```python
from build123d import *

# Parameters (mm, degrees)
SKETCH1_W           = 168
SKETCH1_H           = 112
BOSS_EXTRUDE1_DEPTH = 3
SKETCH2_W           = 23
SKETCH2_H           = 28
BOSS_EXTRUDE2_DEPTH = 81
SKETCH11_W          = 28
SKETCH11_H          = 23
CUT_EXTRUDE4_DEPTH  = 12
SKETCH13_W          = 2.5
SKETCH13_H          = 33.689893656
CUT_EXTRUDE5_DEPTH  = 12
SKETCH17_RX         = 11
SKETCH17_RY         = 10
CUT_EXTRUDE6_DEPTH  = 40
SKETCH18_R          = 17
BOSS_EXTRUDE3_DEPTH = 18
SKETCH19_R          = 14
CUT_EXTRUDE7_DEPTH  = 18
SKETCH20_W          = 20
SKETCH20_H          = 25.807879142
CUT_EXTRUDE8_DEPTH  = 18


with BuildPart() as part:
    # Sketch1 → Boss-Extrude1 (new body)
    with BuildSketch(Plane(origin=(0, 0, 0), x_dir=(1, 0, 0), z_dir=(0, 1, 0))):
        Rectangle(SKETCH1_W, SKETCH1_H)
    extrude(amount=BOSS_EXTRUDE1_DEPTH)

    # Sketch2 → Boss-Extrude2 (add)
    with BuildSketch(Plane(origin=(0, 3, 0), x_dir=(1, 0, 0), z_dir=(0, 1, 0))):
        with Locations((-56.5, 30.5)):
            Rectangle(SKETCH2_W, SKETCH2_H)
    boss_extrude2 = extrude(amount=BOSS_EXTRUDE2_DEPTH)

    # Mirror1: Boss-Extrude2 across plane
    add(boss_extrude2.mirror(Plane(origin=(0, 0, 0), x_dir=(0, 0, 1), z_dir=(1, 0, 0))))

    # Sketch11 → Cut-Extrude4 (cut)
    with BuildSketch(Plane(origin=(0, 84, 0), x_dir=(1, 0, 0), z_dir=(0, 1, 0))):
        with Locations((-59, 30.5)):
            Rectangle(SKETCH11_W, SKETCH11_H)
    extrude(amount=-CUT_EXTRUDE4_DEPTH, mode=Mode.SUBTRACT)

    # Sketch13 → Cut-Extrude5 (cut)
    with BuildSketch(Plane(origin=(0, 72, 0), x_dir=(1, 0, 0), z_dir=(0, 1, 0))):
        with Locations((-50, 30.5)):
            Rectangle(SKETCH13_W, SKETCH13_H)
    extrude(amount=CUT_EXTRUDE5_DEPTH, mode=Mode.SUBTRACT)

    # Sketch17 → Cut-Extrude6 (cut)
    with BuildSketch(Plane.ZY.offset(-45)):
        with Locations((-30.5, 84)):
            Ellipse(SKETCH17_RX, SKETCH17_RY)
    extrude(amount=-CUT_EXTRUDE6_DEPTH, mode=Mode.SUBTRACT)

    # Sketch18 → Boss-Extrude3 (add)
    with BuildSketch(Plane(origin=(0, 3, 0), x_dir=(1, 0, 0), z_dir=(0, 1, 0))):
        with Locations(Location((0, -15.5, 0), (0, 0, 90))):
            Circle(SKETCH18_R)
    extrude(amount=BOSS_EXTRUDE3_DEPTH)

    # Sketch19 → Cut-Extrude7 (cut)
    with BuildSketch(Plane(origin=(0, 21, 0), x_dir=(1, 0, 0), z_dir=(0, 1, 0))):
        with Locations(Location((0, -15.5, 0), (0, 0, 270))):
            Circle(SKETCH19_R)
    extrude(amount=-CUT_EXTRUDE7_DEPTH, mode=Mode.SUBTRACT)

    # Sketch20 → Cut-Extrude8 (cut)
    with BuildSketch(Plane(origin=(0, 21, 0), x_dir=(1, 0, 0), z_dir=(0, 1, 0))):
        with Locations((0, -32.5)):
            Rectangle(SKETCH20_W, SKETCH20_H)
    extrude(amount=-CUT_EXTRUDE8_DEPTH, mode=Mode.SUBTRACT)


solid = part.part
```
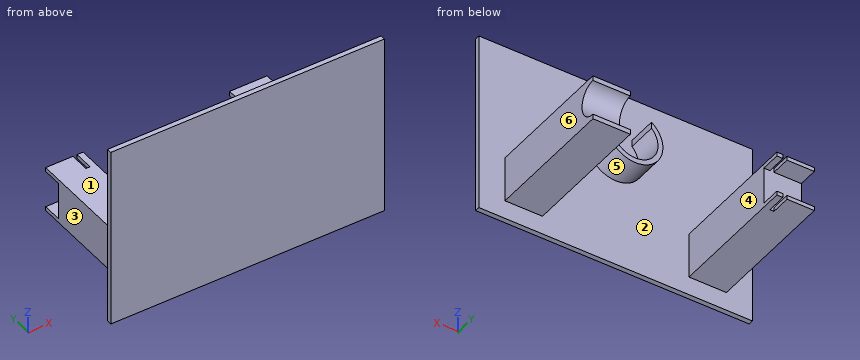
Read the model definition and answer for the solid it produces. Units are mm, in the model's axes. Face numbers are marked on the shaded views. A direction names the side the tool comes from. Round coordinates to 2 decimals unless told otherwise and drop trailing zeros. Write each loop counter-clockwise with the first axis right and the second up, starting at its lowest first coordinate (ties: lowest second). Pieces come first, ordered by that corner, then holes. Notation, with made-up numbers: (-26.5, 65) -> (13.5, 65) arc R26 ccw to (13.5, 101) -> close; hole circle Ø5 at (48, 61.25). An arc over 180 degrees is marked (long way). Answer in a Markdown table with one row per item. Add a question column.
1) Find section B-B, the plane y = 34. Determine the outline of the cut face in (x, z).
2) Find section C-C, the plane z = 15.5. Determine the outline of the cut face in (x, y), and give its area (3 significant figures).
3) Consider line 1 (X direction, y = 62.5, z = -38); line 2 (X direction, y = 12.75, z = 15.5); line 3 (Z direction, x = -65, y = 17). Determine where each line is inside the solid, lowest interval first.
4) Which of the six approach directions +Z, -Z, +X, -X, +Y, -Y give full straight-line access (tool end or side, diameter ignored) to the marked faces 4, 5 and 6?
5) Determine the mould class of the marked faces 1, 2 and 3 for opening direction X: pulls with the +X half, pulls with the -X half, needs draft (parallel to the pull), parting line crosses it, or undercut.
6) Find section D-D, the plane x = -56. Determine the outline of the cut face in (y, z), and give its area (3 significant figures).
7) Given P1, Ø11.5, axis at x = -55.5, y = 31, coming from the +Z side; P2, Ø12, axis at x = -31.5, z = -22.5, coming from the +Y side; P3, Ø0.8, axis at y = 75.5, z = -43, coming from the +X side, each flat-ended and moving along its own axis, determine where each tip first touches the part or whether it passes through.
8) Find section A-A, the plane y = 17. Determine the outline of the cut face in (x, z).
Findings below:
| question | item | result |
|---|---|---|
| 1 | outline | (-68, -44.5) -> (-45, -44.5) -> (-45, -16.5) -> (-68, -16.5) -> close; (45, -44.5) -> (68, -44.5) -> (68, -16.5) -> (45, -16.5) -> close |
| 2 | outline | (-84, 0) -> (84, 0) -> (84, 3) -> (17, 3) -> (17, 21) -> (14, 21) -> (14, 3) -> (-14, 3) -> (-14, 21) -> (-17, 21) -> (-17, 3) -> (-84, 3) -> close |
| 2 | area | 612 mm² |
| 3 | line 1 | -68 to -45, 45 to 68 |
| 3 | line 2 | -17 to -14, 14 to 17 |
| 3 | line 3 | -44.5 to -16.5 |
| 4 | face 4 | +Z, -Z, +Y |
| 4 | face 5 | +Y |
| 4 | face 6 | +Z, -Z, +X, +Y |
| 5 | face 1 | needs draft |
| 5 | face 2 | undercut |
| 5 | face 3 | pulls with the -X half |
| 6 | outline | (0, -56) -> (3, -56) -> (3, -44.5) -> (84, -44.5) -> (84, -42) -> (72, -42) -> (72, -19) -> (84, -19) -> (84, -16.5) -> (3, -16.5) -> (3, 56) -> (0, 56) -> close |
| 6 | area | 2,330 mm² |
| 7 | P1 | z = -16.5 |
| 7 | P2 | y = 3 |
| 7 | P3 | x = 68 |
| 8 | outline | (-68, -44.5) -> (-45, -44.5) -> (-45, -16.5) -> (-68, -16.5) -> close; (-10, 25.3) -> (-10, 29.25) arc R17 ccw (long way) to (10, 29.25) -> (10, 25.3) arc R14 cw (long way) to start; (45, -44.5) -> (68, -44.5) -> (68, -16.5) -> (45, -16.5) -> close |
